The listing builds one solid part. Answer for the finished solid, in the listing's coordinates (mm). A direction names the side the tool comes from. Round coordinates to 2 decimals unless told otherwise and drop trailing zeros. Order: outer loops, then holes, each group sorted by start corner. A loop starts at its lowest first (then second) coordinate and runs counter-clockwise, first axis right, second up. Notation, with made-up numbers: (-10.5, 25) -> (14.5, 25) arc R26 ccw to (14.5, 44) -> close; hole circle Ø6 at (-30, 21). An arc over 180 degrees is marked (long way). Answer in a Markdown table with one row per item. Add a question column.
```python
from build123d import *

# Parameters (mm, degrees)
F0_W     = 76.2
F0_H     = 76.2
F1_DEPTH = 12.7
F2_DEPTH = 50.8
F3_DEPTH = 12.7


with BuildPart() as f1:
    # F0 (on Top) → F1 (new body)
    with BuildSketch(Plane.XY):
        Rectangle(F0_W, F0_H)
        with BuildLine():
            Line((30.565725, -32.5501), (-30.565725, -32.5501))
            ThreePointArc((-30.565725, -32.5501), (-33.9532650189, -33.9532650189), (-32.5501, -30.565725))
            Line((-32.5501, -30.565725), (-32.5501, 30.565725))
            ThreePointArc((-32.5501, 30.565725), (-33.9532650189, 33.9532650189), (-30.565725, 32.5501))
            Line((-30.565725, 32.5501), (30.565725, 32.5501))
            ThreePointArc((30.565725, 32.5501), (32.5501, 34.534475), (34.534475, 32.5501))
            ThreePointArc((34.534475, 32.5501), (33.9532650189, 31.1469349811), (32.5501, 30.565725))
            Line((32.5501, 30.565725), (32.5501, -30.565725))
            ThreePointArc((32.5501, -30.565725), (33.9532650189, -31.1469349811), (34.534475, -32.5501))
            ThreePointArc((34.534475, -32.5501), (32.5501, -34.534475), (30.565725, -32.5501))
        make_face(mode=Mode.SUBTRACT)
        with BuildLine():
            ThreePointArc((-31.75, -30.7341748554), (-31.1469349811, -31.1469349811), (-30.7341748554, -31.75))
            Line((-30.7341748554, -31.75), (30.7341748554, -31.75))
            ThreePointArc((30.7341748554, -31.75), (31.1469349811, -31.1469349811), (31.75, -30.7341748554))
            Line((31.75, -30.7341748554), (31.75, 30.7341748554))
            ThreePointArc((31.75, 30.7341748554), (31.1469349811, 31.1469349811), (30.7341748554, 31.75))
            Line((30.7341748554, 31.75), (-30.7341748554, 31.75))
            ThreePointArc((-30.7341748554, 31.75), (-31.1469349811, 31.1469349811), (-31.75, 30.7341748554))
            Line((-31.75, 30.7341748554), (-31.75, -30.7341748554))
        make_face()
        with BuildLine():
            ThreePointArc((31.75, -30.7341748554), (32.1412799406, -30.6082940623), (32.5501, -30.565725))
            Line((32.5501, -30.565725), (32.5501, 30.565725))
            ThreePointArc((32.5501, 30.565725), (32.1412799406, 30.6082940623), (31.75, 30.7341748554))
            Line((31.75, 30.7341748554), (31.75, -30.7341748554))
        make_face()
        with BuildLine():
            ThreePointArc((-30.7341748554, -31.75), (-30.6082940623, -32.1412799406), (-30.565725, -32.5501))
            Line((-30.565725, -32.5501), (30.565725, -32.5501))
            ThreePointArc((30.565725, -32.5501), (30.6082940623, -32.1412799406), (30.7341748554, -31.75))
            Line((30.7341748554, -31.75), (-30.7341748554, -31.75))
        make_face()
        with BuildLine():
            Line((30.565725, 32.5501), (-30.565725, 32.5501))
            ThreePointArc((-30.565725, 32.5501), (-30.6082940623, 32.1412799406), (-30.7341748554, 31.75))
            Line((-30.7341748554, 31.75), (30.7341748554, 31.75))
            ThreePointArc((30.7341748554, 31.75), (30.6082940623, 32.1412799406), (30.565725, 32.5501))
        make_face()
        with BuildLine():
            Line((-32.5501, 30.565725), (-32.5501, -30.565725))
            ThreePointArc((-32.5501, -30.565725), (-32.1412799406, -30.6082940623), (-31.75, -30.7341748554))
            Line((-31.75, -30.7341748554), (-31.75, 30.7341748554))
            ThreePointArc((-31.75, 30.7341748554), (-32.1412799406, 30.6082940623), (-32.5501, 30.565725))
        make_face()
        with BuildLine():
            ThreePointArc((-32.5501, -30.565725), (-33.9532650189, -33.9532650189), (-30.565725, -32.5501))
            Line((-30.565725, -32.5501), (-32.5501, -32.5501))
            Line((-32.5501, -32.5501), (-32.5501, -30.565725))
        make_face()
        with BuildLine():
            Line((32.5501, 32.5501), (32.5501, 30.565725))
            ThreePointArc((32.5501, 30.565725), (33.9532650189, 31.1469349811), (34.534475, 32.5501))
            ThreePointArc((34.534475, 32.5501), (32.5501, 34.534475), (30.565725, 32.5501))
            Line((30.565725, 32.5501), (32.5501, 32.5501))
        make_face()
        with BuildLine():
            ThreePointArc((-30.565725, 32.5501), (-33.9532650189, 33.9532650189), (-32.5501, 30.565725))
            Line((-32.5501, 30.565725), (-32.5501, 32.5501))
            Line((-32.5501, 32.5501), (-30.565725, 32.5501))
        make_face()
        with BuildLine():
            Line((32.5501, -32.5501), (30.565725, -32.5501))
            ThreePointArc((30.565725, -32.5501), (32.5501, -34.534475), (34.534475, -32.5501))
            ThreePointArc((34.534475, -32.5501), (33.9532650189, -31.1469349811), (32.5501, -30.565725))
            Line((32.5501, -30.565725), (32.5501, -32.5501))
        make_face()
        with BuildLine():
            ThreePointArc((31.75, 30.7341748554), (32.1412799406, 30.6082940623), (32.5501, 30.565725))
            Line((32.5501, 30.565725), (32.5501, 32.5501))
            Line((32.5501, 32.5501), (30.565725, 32.5501))
            ThreePointArc((30.565725, 32.5501), (30.6082940623, 32.1412799406), (30.7341748554, 31.75))
            Line((30.7341748554, 31.75), (31.75, 31.75))
            Line((31.75, 31.75), (31.75, 30.7341748554))
        make_face()
        with BuildLine():
            Line((-32.5501, -32.5501), (-30.565725, -32.5501))
            ThreePointArc((-30.565725, -32.5501), (-30.6082940623, -32.1412799406), (-30.7341748554, -31.75))
            Line((-30.7341748554, -31.75), (-31.75, -31.75))
            Line((-31.75, -31.75), (-31.75, -30.7341748554))
            ThreePointArc((-31.75, -30.7341748554), (-32.1412799406, -30.6082940623), (-32.5501, -30.565725))
            Line((-32.5501, -30.565725), (-32.5501, -32.5501))
        make_face()
        with BuildLine():
            Line((-31.75, 31.75), (-31.75, 30.7341748554))
            ThreePointArc((-31.75, 30.7341748554), (-31.1469349811, 31.1469349811), (-30.7341748554, 31.75))
            Line((-30.7341748554, 31.75), (-31.75, 31.75))
        make_face()
        with BuildLine():
            ThreePointArc((30.7341748554, -31.75), (30.6082940623, -32.1412799406), (30.565725, -32.5501))
            Line((30.565725, -32.5501), (32.5501, -32.5501))
            Line((32.5501, -32.5501), (32.5501, -30.565725))
            ThreePointArc((32.5501, -30.565725), (32.1412799406, -30.6082940623), (31.75, -30.7341748554))
            Line((31.75, -30.7341748554), (31.75, -31.75))
            Line((31.75, -31.75), (30.7341748554, -31.75))
        make_face()
        with BuildLine():
            ThreePointArc((30.7341748554, 31.75), (31.1469349811, 31.1469349811), (31.75, 30.7341748554))
            Line((31.75, 30.7341748554), (31.75, 31.75))
            Line((31.75, 31.75), (30.7341748554, 31.75))
        make_face()
        with BuildLine():
            Line((-31.75, -31.75), (-30.7341748554, -31.75))
            ThreePointArc((-30.7341748554, -31.75), (-31.1469349811, -31.1469349811), (-31.75, -30.7341748554))
            Line((-31.75, -30.7341748554), (-31.75, -31.75))
        make_face()
        with BuildLine():
            ThreePointArc((31.75, -30.7341748554), (31.1469349811, -31.1469349811), (30.7341748554, -31.75))
            Line((30.7341748554, -31.75), (31.75, -31.75))
            Line((31.75, -31.75), (31.75, -30.7341748554))
        make_face()
        with BuildLine():
            Line((-32.5501, 32.5501), (-32.5501, 30.565725))
            ThreePointArc((-32.5501, 30.565725), (-32.1412799406, 30.6082940623), (-31.75, 30.7341748554))
            Line((-31.75, 30.7341748554), (-31.75, 31.75))
            Line((-31.75, 31.75), (-30.7341748554, 31.75))
            ThreePointArc((-30.7341748554, 31.75), (-30.6082940623, 32.1412799406), (-30.565725, 32.5501))
            Line((-30.565725, 32.5501), (-32.5501, 32.5501))
        make_face()
    extrude(amount=-F1_DEPTH)

    # F0 (on Top) → F2 (join)
    with BuildSketch(Plane.XY):
        with BuildLine():
            ThreePointArc((-31.75, -30.7341748554), (-31.1469349811, -31.1469349811), (-30.7341748554, -31.75))
            Line((-30.7341748554, -31.75), (30.7341748554, -31.75))
            ThreePointArc((30.7341748554, -31.75), (31.1469349811, -31.1469349811), (31.75, -30.7341748554))
            Line((31.75, -30.7341748554), (31.75, 30.7341748554))
            ThreePointArc((31.75, 30.7341748554), (31.1469349811, 31.1469349811), (30.7341748554, 31.75))
            Line((30.7341748554, 31.75), (-30.7341748554, 31.75))
            ThreePointArc((-30.7341748554, 31.75), (-31.1469349811, 31.1469349811), (-31.75, 30.7341748554))
            Line((-31.75, 30.7341748554), (-31.75, -30.7341748554))
        make_face()
    extrude(amount=F2_DEPTH)

    # F0 (on Top) → F3 (cut, through all)
    with BuildSketch(Plane.XY):
        with BuildLine():
            ThreePointArc((-32.5501, -30.565725), (-33.9532650189, -33.9532650189), (-30.565725, -32.5501))
            Line((-30.565725, -32.5501), (-32.5501, -32.5501))
            Line((-32.5501, -32.5501), (-32.5501, -30.565725))
        make_face()
        with BuildLine():
            Line((-32.5501, -32.5501), (-30.565725, -32.5501))
            ThreePointArc((-30.565725, -32.5501), (-30.6082940623, -32.1412799406), (-30.7341748554, -31.75))
            Line((-30.7341748554, -31.75), (-31.75, -31.75))
            Line((-31.75, -31.75), (-31.75, -30.7341748554))
            ThreePointArc((-31.75, -30.7341748554), (-32.1412799406, -30.6082940623), (-32.5501, -30.565725))
            Line((-32.5501, -30.565725), (-32.5501, -32.5501))
        make_face()
        with BuildLine():
            Line((-31.75, -31.75), (-30.7341748554, -31.75))
            ThreePointArc((-30.7341748554, -31.75), (-31.1469349811, -31.1469349811), (-31.75, -30.7341748554))
            Line((-31.75, -30.7341748554), (-31.75, -31.75))
        make_face()
        with BuildLine():
            Line((32.5501, -32.5501), (30.565725, -32.5501))
            ThreePointArc((30.565725, -32.5501), (32.5501, -34.534475), (34.534475, -32.5501))
            ThreePointArc((34.534475, -32.5501), (33.9532650189, -31.1469349811), (32.5501, -30.565725))
            Line((32.5501, -30.565725), (32.5501, -32.5501))
        make_face()
        with BuildLine():
            ThreePointArc((30.7341748554, -31.75), (30.6082940623, -32.1412799406), (30.565725, -32.5501))
            Line((30.565725, -32.5501), (32.5501, -32.5501))
            Line((32.5501, -32.5501), (32.5501, -30.565725))
            ThreePointArc((32.5501, -30.565725), (32.1412799406, -30.6082940623), (31.75, -30.7341748554))
            Line((31.75, -30.7341748554), (31.75, -31.75))
            Line((31.75, -31.75), (30.7341748554, -31.75))
        make_face()
        with BuildLine():
            ThreePointArc((31.75, -30.7341748554), (31.1469349811, -31.1469349811), (30.7341748554, -31.75))
            Line((30.7341748554, -31.75), (31.75, -31.75))
            Line((31.75, -31.75), (31.75, -30.7341748554))
        make_face()
        with BuildLine():
            ThreePointArc((30.7341748554, 31.75), (31.1469349811, 31.1469349811), (31.75, 30.7341748554))
            Line((31.75, 30.7341748554), (31.75, 31.75))
            Line((31.75, 31.75), (30.7341748554, 31.75))
        make_face()
        with BuildLine():
            ThreePointArc((31.75, 30.7341748554), (32.1412799406, 30.6082940623), (32.5501, 30.565725))
            Line((32.5501, 30.565725), (32.5501, 32.5501))
            Line((32.5501, 32.5501), (30.565725, 32.5501))
            ThreePointArc((30.565725, 32.5501), (30.6082940623, 32.1412799406), (30.7341748554, 31.75))
            Line((30.7341748554, 31.75), (31.75, 31.75))
            Line((31.75, 31.75), (31.75, 30.7341748554))
        make_face()
        with BuildLine():
            Line((32.5501, 32.5501), (32.5501, 30.565725))
            ThreePointArc((32.5501, 30.565725), (33.9532650189, 31.1469349811), (34.534475, 32.5501))
            ThreePointArc((34.534475, 32.5501), (32.5501, 34.534475), (30.565725, 32.5501))
            Line((30.565725, 32.5501), (32.5501, 32.5501))
        make_face()
        with BuildLine():
            ThreePointArc((-30.565725, 32.5501), (-33.9532650189, 33.9532650189), (-32.5501, 30.565725))
            Line((-32.5501, 30.565725), (-32.5501, 32.5501))
            Line((-32.5501, 32.5501), (-30.565725, 32.5501))
        make_face()
        with BuildLine():
            Line((-32.5501, 32.5501), (-32.5501, 30.565725))
            ThreePointArc((-32.5501, 30.565725), (-32.1412799406, 30.6082940623), (-31.75, 30.7341748554))
            Line((-31.75, 30.7341748554), (-31.75, 31.75))
            Line((-31.75, 31.75), (-30.7341748554, 31.75))
            ThreePointArc((-30.7341748554, 31.75), (-30.6082940623, 32.1412799406), (-30.565725, 32.5501))
            Line((-30.565725, 32.5501), (-32.5501, 32.5501))
        make_face()
        with BuildLine():
            Line((-31.75, 31.75), (-31.75, 30.7341748554))
            ThreePointArc((-31.75, 30.7341748554), (-31.1469349811, 31.1469349811), (-30.7341748554, 31.75))
            Line((-30.7341748554, 31.75), (-31.75, 31.75))
        make_face()
    extrude(amount=-F3_DEPTH, mode=Mode.SUBTRACT)


solid = f1.part
```
1. Straight lines are drawn through the part: line 1 along X through (y, z) = (-30.5, 38); line 2 along Z through (x, y) = (35, -4). For each, find the intervals that lie inside material, in ascending order.
2. The part is cut by section B-B (x = -17.5). Give the vertices of the cut face in (y, z), then the cut area to 3 significant figures.
3. The part is cut by section A-A (z = 17.5). Give the vertices of the cut face in (x, y).
4. For faces 1 (the flat face through (31.75, 0, 25)), 2 (the flat face through (-34, 1, 0)), 3 (the flat face through (0, -31.75, 25)), 4 (the flat face through (-31.75, 0, 25)), 5 (the flat face through (0, 31.75, 25)), determine the directions among +Z, -Z, +X, -X, +Y, -Y from which every point of the face is accessible in a straight line to the end or side of a thin tool.
5. Each of these flat-tipped pins is pushed along its axis until it touches: pin 1 (3 mm diameter, centred on x = -32.55, y = -32.55, fed in from +Z); pin 2 (1 mm diameter, centred on x = -18, z = 25.5, fed in from +Y); pin 3 (12 mm diameter, centred on x = -0.5, z = 33.5, fed in from -Y); pin 4 (15 mm diameter, centred on y = 12.5, z = 32, fed in from -X). Where does it stop, or does it pass through?
Report:
| question | item | result |
|---|---|---|
| 1 | line 1 | x = -31.75 to 31.75 |
| 1 | line 2 | z = -12.7 to 0 |
| 2 | outline | (-38.1, -12.7) -> (38.1, -12.7) -> (38.1, 0) -> (31.75, 0) -> (31.75, 50.8) -> (-31.75, 50.8) -> (-31.75, 0) -> (-38.1, 0) -> close |
| 2 | area | 4,190 mm^2 |
| 3 | outline | (-31.75, -30.73) arc R1.98 cw to (-30.73, -31.75) -> (30.73, -31.75) arc R1.98 cw to (31.75, -30.73) -> (31.75, 30.73) arc R1.98 cw to (30.73, 31.75) -> (-30.73, 31.75) arc R1.98 cw to (-31.75, 30.73) -> close |
| 4 | face 1 | +Z, +X, +Y, -Y |
| 4 | face 2 | +Z |
| 4 | face 3 | +Z, +X, -X, -Y |
| 4 | face 4 | +Z, -X, +Y, -Y |
| 4 | face 5 | +Z, +X, -X, +Y |
| 5 | pin 1 | passes through |
| 5 | pin 2 | stops at y = 31.75 |
| 5 | pin 3 | stops at y = -31.75 |
| 5 | pin 4 | stops at x = -31.75 |
